Job drawing, mm, ordinate dimensions from the low corner. One solid piece. A direction names the side the tool comes from. Round coordinates to 2 decimals unless told otherwise and drop trailing zeros. Order: outer loops, then holes, each group sorted by start corner. A loop starts at its lowest first (then second) coordinate and runs counter-clockwise, first axis right, second up. Notation, with made-up numbers: (1, -29) - (12, -29) arc R9 ccw to (12, -13) - close; hole circle Ø1 at (-9, 2.25). An arc over 180 degrees is marked (long way). Use one line per item in the form item = value. Start each with the question number.
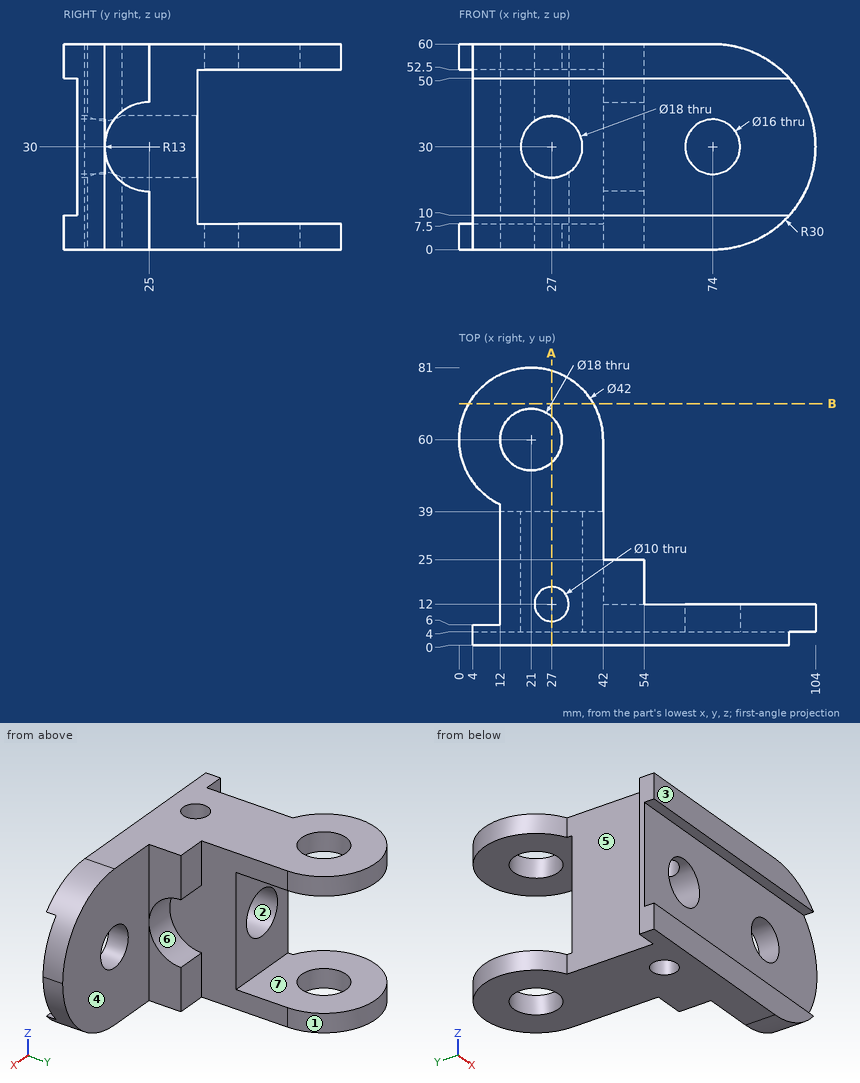
(1) Wall check: line 1 (Y direction, x = 27, z = 13.75); line 2 (Z direction, x = 27, y = 18); line 3 (Z direction, x = 10.5, y = 77.5). Give the ranges that are in metal, low to high. Write a range as [from, to].
(2) Mould opens along X. For the marked faces 1, 2 and 3 say: pulls with the +X half, pulls with the -X half, needs draft (parallel to the pull), parting line crosses it, or undercut.
(3) Which spindle directions (+Z, -Z, +X, -X, +Y, -Y) get a long thin tool onto all of the face, cutting with end or side? Do the marked faces 4, 5, 6 and 7. Say none if no direction does.
(4) Slice it at B-B (y = 70.5). Give the cut face in (x, z).
(5) Slice it at A-A (x = 27). Give the number of separate pieces and of enclosed holes in the cut face, and give its area (3 significant figures).
(6) Flat gauge pins, fed straight in: P1, Ø4, axis at y = 30, z = 17, coming from the -X side; P2, Ø6.5, axis at y = 16.5, z = 51.5, coming from the +X side; P3, Ø2.5, axis at x = 9, z = 36.5, coming from the +Y side. Where does each tip first touch, or does it go through?
Results list:
q1.line_1 = [4, 7], [17, 39]
q1.line_2 = [0, 21], [39, 60]
q1.line_3 = [0, 7.5], [52.5, 60]
q2.face_1 = parting line crosses it
q2.face_2 = undercut
q2.face_3 = needs draft
q3.face_4 = +Z, -Z, +X, +Y
q3.face_5 = +Z, -Z, -X
q3.face_6 = +X, +Y
q3.face_7 = +X, -X, +Y
q4.outline = (2.81, 0) - (39.19, 0) - (39.19, 7.5) - (2.81, 7.5) - close; (2.81, 52.5) - (39.19, 52.5) - (39.19, 60) - (2.81, 60) - close
q5.separate_pieces = 6
q5.enclosed_holes = 0
q5.area = 1,550 mm²
q6.P1 = 12
q6.P2 = 54
q6.P3 = 6
